Geometry: final body of the model. Coordinates: model frame, mm. A direction names the side the tool comes from. Round coordinates to 2 decimals unless told otherwise and drop trailing zeros. Write each loop counter-clockwise with the first axis right and the second up, starting at its lowest first coordinate (ties: lowest second). Pieces come first, ordered by that corner, then holes. Notation, with made-up numbers: M 87,-9.75 L 137,-9.75 A14 cw 137,0.25 Z; hole C 6,12.25 d1. An arc over 180 degrees is marked long. Use one line per item in the form item = value. Start each with the question number.
Item 1: Section query A-A (x = 0). Return loops of the section in (y, z), and give its area (3 significant figures).
Item 2: Section query C-C (y = -10.5). Return loops of the section in (x, z), and give its area (3 significant figures).
Item 3: Section query B-B (z = 5). Return loops of the section in (x, y), and give its area (3 significant figures).
Item 4: Pin query (flat end, axial travel): pin 1 Ø1 at (x, z) = (-10.5, -42.5) entering from +Y; pin 2 Ø12 at (x, z) = (48, -4) entering from -Y; pin 3 Ø4 at (y, z) = (-32, -25.5) entering from +X. Return the tip coordinate at first contact, or that it passes through.
Item 5: Ray query, probe 1 along Y at (x, z) = (28, -1); probe 2 along X at (y, z) = (-36, 0); probe 3 along Z at (x, y) = (-8.5, -11). Return the intervals inside material, ascending.
Item 6: Reachability of faces 1 (the flat face through (-29, -50.8, -13)), 2 (the flat face through (15.359, -37.922, -39.332)) from +Z, -Z, +X, -X, +Y, -Y: full face, straight path, thin tool, end or side. Return the list, or none.
Item 7: Section query D-D (y = -28.5). Return loops of the section in (x, z), and give its area (3 significant figures).
from build123d import *

# Parameters (mm, degrees)
F0_W     = 124.46073
F0_H     = 108.976554
F1_DEPTH = 25.4
F3_DEPTH = 25.4
F5_DEPTH = 50.801


with BuildPart() as f1:
    # F0 (on Front) → F1 (new body)
    with BuildSketch(Plane.XZ):
        with Locations((0.717355, -1.765637)):
            Rectangle(F0_W, F0_H)
    extrude(amount=F1_DEPTH)

    # F2 (on face) → F3 (join)
    with BuildSketch(Plane.XZ.offset(25.4)):
        Polygon((22.376237, -56.253914), (-22.816991, 52.72264), (-61.51301, 52.72264), (-61.51301, -56.253914), align=None)
    extrude(amount=F3_DEPTH)

    # F4 (on face) → F5 (cut, through all)
    with BuildSketch(Plane.XZ.offset(50.8)):
        with BuildLine():
            ThreePointArc((8.141664, -21.929417), (19.204633, -13.355452), (23.392008, 0))
            ThreePointArc((23.392008, 0), (12.623583, 19.69343), (-9.767282, 21.255264))
            Line((-9.767282, 21.255264), (8.141664, -21.929417))
        make_face()
        with BuildLine():
            Line((8.141664, -21.929417), (-9.767282, 21.255264))
            ThreePointArc((-9.767282, 21.255264), (-21.607634, -8.960815), (8.141664, -21.929417))
        make_face()
    extrude(amount=-F5_DEPTH, mode=Mode.SUBTRACT)


solid = f1.part
Working result:
q1.outline = M -50.8,-56.25 L 0,-56.25 L 0,-23.39 L -50.8,-23.39 Z; M -25.4,23.39 L 0,23.39 L 0,52.72 L -25.4,52.72 Z
q1.area = 2,410 mm²
q2.outline = M -61.51,-56.25 L 62.95,-56.25 L 62.95,52.72 L -61.51,52.72 Z; hole C 0,0 d46.78
q2.area = 11,800 mm²
q3.outline = M -61.51,-50.8 L -22.85,-50.8 L -22.85,0 L -61.51,0 Z; M 22.85,-25.4 L 62.95,-25.4 L 62.95,0 L 22.85,0 Z
q3.area = 2,980 mm²
q4.pin_1 = 0
q4.pin_2 = -25.4
q4.pin_3 = 10.45
q5.probe_1 = -25.4 to 0
q5.probe_2 = -61.51 to -23.39
q5.probe_3 = -56.25 to -21.79, 21.79 to 52.72
q6.face_1 = +Z, -Z, +X, -X, -Y
q6.face_2 = +Z, +X, -Y
q7.outline = M -61.51,-56.25 L 22.38,-56.25 L 8.14,-21.93 A23.39 cw -9.77,21.26 L -22.82,52.72 L -61.51,52.72 Z
q7.area = 5,860 mm²
